Read the model definition and answer for the solid it produces. Units are mm, in the model's axes. A direction names the side the tool comes from. Give positions to 0.01 mm unless a question says otherwise; leave off trailing zeros. Write each loop counter-clockwise with the first axis right and the second up, starting at its lowest first coordinate (ties: lowest second). Pieces come first, ordered by that corner, then holes. Notation, with made-up numbers: M -3,58 L 19,58 A26 ccw 19,81 Z; hole C -32.75,23 d1. An arc over 180 degrees is marked long. Use a Markdown table: item, result. Add a question column.
Item 1: A cutting plane is placed at C-C on z = 0. Determine the outline of the cut face in (x, y).
Item 2: Given P1, Ø2, axis at y = 25, z = -10.5, coming from the +X side; P2, Ø12, axis at x = -0.5, z = -2, coming from the -Y side; P3, Ø1.5, axis at y = 29.5, z = -8, coming from the +X side; P4, Ø3, axis at x = -0.5, y = 31.5, coming from the -Z side, each flat-ended and moving along its own axis, determine where each tip first touches the part or whether it passes through.
Item 3: Consider probe 1 along X at (y, z) = (42.55, 0); probe 2 along Z at (x, y) = (-4, 42.5); probe 3 along Z at (x, y) = (0, 31). Determine where each line is inside the solid, lowest interval first. Write a range as [from, to].
Item 4: A cutting plane is placed at D-D on y = 17.5. Determine the outline of the cut face in (x, z).
Item 5: A cutting plane is placed at A-A on y = 41.5. Determine the outline of the cut face in (x, z), then the cut area to 3 significant figures.
Item 6: For faces 1 (the flat face through (-2.5, 41, 5.2)), 2 (the cylindrical face through (4.88, 24.32, -1.08)), 3 (the cylindrical face through (-3.604, 0.986, 11.446)), 4 (the flat face through (7, 21, -12)), determine the directions among +Z, -Z, +X, -X, +Y, -Y from which every point of the face is accessible in a straight line to the end or side of a thin tool.
Item 7: A cutting plane is placed at B-B on x = 0. Determine the outline of the cut face in (y, z), then the cut area to 3 significant figures.
from build123d import *

# Parameters (mm, degrees)
SKETCH1_R         = 12.5
ENCLOSURE_DEPTH   = 41
SKETCH3_R         = 12.5
SKETCH3_R_2       = 12
UPPER_LIP_DEPTH   = 2
SKETCH4_R         = 5.5
UPPER_SHAFT_DEPTH = 6
SKETCH5_R         = 5
CENTRAL_CUT_DEPTH = 51.214539727
SKETCH6_R         = 12
LOWER_LIP_DEPTH   = 2
SKETCH7_R         = 5.5
SKETCH7_R_2       = 5
LOWER_SHAFT_DEPTH = 1
FILM_START        = -43
FILM_LIP_DEPTH    = 43


with BuildPart() as part:
    # Sketch1 → Enclosure (new body)
    with BuildSketch(Plane(origin=(0, 0, 0), x_dir=(1, 0, 0), z_dir=(0, 1, 0))):
        with Locations(Location((0, 0, 0), (0, 0, 270))):
            Circle(SKETCH1_R)
    extrude(amount=ENCLOSURE_DEPTH)

    # Sketch3 → Upper Lip (add)
    with BuildSketch(Plane(origin=(0, 41, 0), x_dir=(1, 0, 0), z_dir=(0, 1, 0))):
        with Locations(Location((0, 0, 0), (0, 0, 270))):
            Circle(SKETCH3_R)
        with Locations(Location((0, 0, 0), (0, 0, 270))):
            Circle(SKETCH3_R_2, mode=Mode.SUBTRACT)
    extrude(amount=UPPER_LIP_DEPTH)

    # Sketch4 → Upper Shaft (add)
    with BuildSketch(Plane(origin=(0, 41, 0), x_dir=(1, 0, 0), z_dir=(0, 1, 0))):
        with Locations(Location((0, 0, 0), (0, 0, 270))):
            Circle(SKETCH4_R)
    extrude(amount=UPPER_SHAFT_DEPTH)

    # Sketch5 → Central Cut (cut, through all)
    with BuildSketch(Plane(origin=(0, 47, 0), x_dir=(1, 0, 0), z_dir=(0, 1, 0))):
        with Locations(Location((0, 0, 0), (0, 0, 270))):
            Circle(SKETCH5_R)
    extrude(amount=-CENTRAL_CUT_DEPTH, mode=Mode.SUBTRACT)

    # Sketch6 → Lower Lip (cut)
    with BuildSketch(Plane.XZ):
        with Locations(Location((0, 0, 0), (0, 0, 90))):
            Circle(SKETCH6_R)
    extrude(amount=-LOWER_LIP_DEPTH, mode=Mode.SUBTRACT)

    # Sketch7 → Lower Shaft (add)
    with BuildSketch(Plane(origin=(0, 2, 0), x_dir=(-1, 0, 0), z_dir=(0, -1, 0))):
        with Locations(Location((0, 0, 0), (0, 0, 270))):
            Circle(SKETCH7_R)
        with Locations(Location((0, 0, 0), (0, 0, 270))):
            Circle(SKETCH7_R_2, mode=Mode.SUBTRACT)
    extrude(amount=LOWER_SHAFT_DEPTH)

    # Sketch8 → Film Lip (add)
    with BuildSketch(Plane(origin=(0, 43, 0), x_dir=(1, 0, 0), z_dir=(0, 1, 0)).offset(FILM_START)):
        with BuildLine():
            Line((3.5, 12), (11.5, 12))
            Line((11.5, 12), (11.5, 10))
            Line((11.5, 10), (7.5, 10))
            ThreePointArc((7.5, 10), (5.590169944, 11.180339887), (3.5, 12))
        make_face()
    extrude(amount=FILM_LIP_DEPTH)


solid = part.part
Filled in:
| question | item | result |
|---|---|---|
| 1 | outline | M -12.5,0 L -12,0 L -12,2 L -5.5,2 L -5.5,1 L -5,1 L -5,47 L -5.5,47 L -5.5,41 L -12,41 L -12,43 L -12.5,43 Z; M 5,1 L 5.5,1 L 5.5,2 L 12,2 L 12,0 L 12.5,0 L 12.5,43 L 12,43 L 12,41 L 5.5,41 L 5.5,47 L 5,47 Z |
| 2 | P1 | x = 11.5 |
| 2 | P2 | y = 1 |
| 2 | P3 | x = 10.18 |
| 2 | P4 | z = -12.5 |
| 3 | probe 1 | [-12.5, -12], [-5.5, -5], [5, 5.5], [12, 12.5] |
| 3 | probe 2 | [-11.84, -11.31], [-3.77, -3], [3, 3.77], [11.31, 11.84] |
| 3 | probe 3 | [-12.5, -5], [5, 12.5] |
| 4 | outline | M 3.5,-12 L 11.5,-12 L 11.5,-10 L 7.5,-10 A12.5 ccw long Z; hole C 0,0 d10 |
| 5 | outline | C 0,0 d11; M 3.5,-12 L 11.5,-12 L 11.5,-10 L 7.5,-10 A12.5 ccw long Z; hole C 0,0 d24; hole C 0,0 d10 |
| 5 | area | 66.4 mm² |
| 6 | face 1 | +Y |
| 6 | face 2 | +Y, -Y |
| 6 | face 3 | -Y |
| 6 | face 4 | -Z, +X, +Y, -Y |
| 7 | outline | M 0,-12.5 L 43,-12.5 L 43,-12 L 41,-12 L 41,-5.5 L 47,-5.5 L 47,-5 L 1,-5 L 1,-5.5 L 2,-5.5 L 2,-12 L 0,-12 Z; M 0,12 L 2,12 L 2,5.5 L 1,5.5 L 1,5 L 47,5 L 47,5.5 L 41,5.5 L 41,12 L 43,12 L 43,12.5 L 0,12.5 Z |
| 7 | area | 596 mm² |
